Verification items for this drawing (mm, ordinates from the low corner). A direction names the side the tool comes from. Coordinates: 2 decimals unless noted, no trailing zeros. Write each loop counter-clockwise with the first axis right and the second up, starting at its lowest first coordinate (ties: lowest second). Pieces come first, ordered by that corner, then holes. Notation, with made-up numbers: M 10.5,33 L 62.5,33 A32 ccw 62.5,71 Z; hole C 52,79.5 d9. An arc over 180 degrees is marked long. Write each question's results on one line, items separated by ' | '.
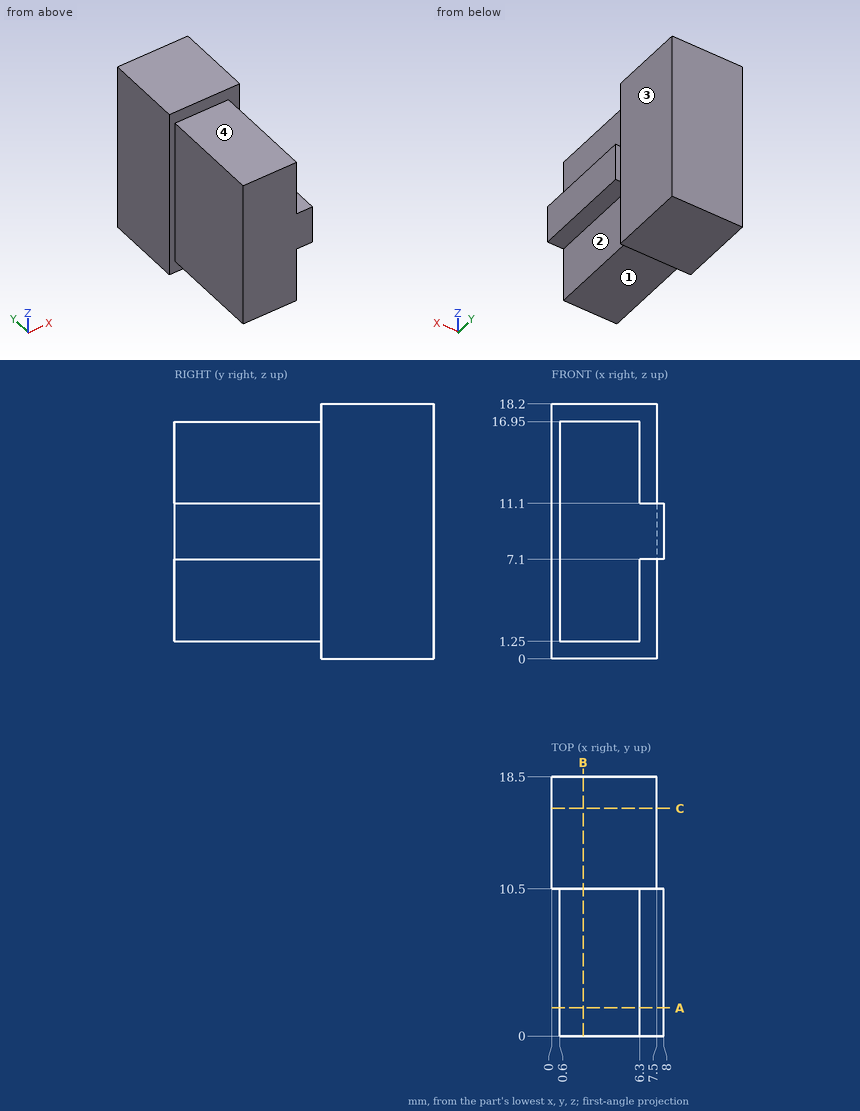
Q1. Sectioned sample at A-A on y = 2. Record the cut outline in (x, z), and give its area (3 significant figures).
Geometry check:
outline: M 0.6,1.25 L 6.3,1.25 L 6.3,7.1 L 8,7.1 L 8,11.1 L 6.3,11.1 L 6.3,16.95 L 0.6,16.95 Z | area: 96.3 mm2
Q2. Access from +Z, -Z, +X, -X, +Y, -Y to the whole of each face (thin tool, end or side, straight path). Record for the marked faces 1, 2, 3 and 4.
Geometry check:
face 1: -Z, +X, -X, -Y | face 2: -Z, +X, -Y | face 3: +Z, -Z, +X, +Y | face 4: +Z, +X, -X, -Y
Q3. Sectioned sample at C-C on y = 16.25. Record the cut outline in (x, z), and give its area (4 significant figures).
Geometry check:
outline: M 0,0 L 7.5,0 L 7.5,18.2 L 0,18.2 Z | area: 136.5 mm2
Q4. Depth check by flat-ended pin: P1, Ø0.8, axis at x = 7, y = 3, coming from the +Z side; P2, Ø6.5, axis at y = 14.5, z = 11.5, coming from the +X side; P3, Ø5, axis at y = 6, z = 7.5, coming from the -X side; P4, Ø2, axis at x = 3.5, z = 12, coming from the -Y side. Enter the tip coordinate at first touch or a pass-through.
Geometry check:
P1: stops at z = 11.1 | P2: stops at x = 7.5 | P3: stops at x = 0.6 | P4: stops at y = 0
Q5. Scan lines: probe 1 along Z at (x, y) = (3.25, 3.5); probe 2 along Z at (x, y) = (6.75, 2.75); probe 3 along Y at (x, z) = (0.5, 3.5). Record each from-to range of solid material in increasing order.
Geometry check:
probe 1: z = 1.25 to 16.95 | probe 2: z = 7.1 to 11.1 | probe 3: y = 10.5 to 18.5
Q6. Sectioned sample at B-B on x = 2.25. Record the cut outline in (y, z).
Geometry check:
outline: M 0,1.25 L 10.5,1.25 L 10.5,0 L 18.5,0 L 18.5,18.2 L 10.5,18.2 L 10.5,16.95 L 0,16.95 Z
